Geometry: final body of the model. Coordinates: model frame, mm. A direction names the side the tool comes from. Give positions to 0.01 mm unless a question says otherwise; leave off trailing zeros. Loops run counter-clockwise (first coordinate to the right, second up) from the corner with the lowest first, then second, coordinate; pieces in that order, holes last. Notation, with made-up numbers: (3, 13.5) -> (37, 13.5) arc R26 cw to (37, 39.5) -> close; hole circle Ø8 at (25.5, -4). An arc over 180 degrees is marked (long way). One line per item, written item: value. Start each with the question number.
Autodesk Inventor part; units mm, degrees
ref_plane "YZ Plane" through (0, 0, 0) normal (1, 0, 0) x (0, 1, 0)
ref_plane "XZ Plane" through (0, 0, 0) normal (0, 1, 0) x (-1, 0, 0)
ref_plane "XY Plane" through (0, 0, 0) normal (0, 0, 1) x (1, 0, 0)
sketch "Sketch1" plane through (0, 0, 0) normal (0, 1, 0) x (-1, 0, 0)
  line L0 (0, 0) -> (80, 0)
  line L1 (80, 0) -> (80, 3.95)
  line L2 (80, 3.95) -> (67, 3.95)
  line L3 (67, 3.95) -> (67, 5)
  line L4 (67, 5) -> (62, 5)
  line L5 (62, 5) -> (62, 6)
  line L6 (62, 6) -> (18, 6)
  line L7 (18, 6) -> (18, 5)
  line L8 (18, 5) -> (13, 5)
  line L9 (13, 5) -> (13, 3.95)
  line L10 (13, 3.95) -> (0, 3.95)
  line L11 (0, 3.95) -> (0, 0)
  point P0 (40, 6)
  dimension "d0" = 80
  dimension "d1" = 3.95
  dimension "d2" = 18
  dimension "d3" = 5
  dimension "d4" = 5
  dimension "d5" = 6
  dimension "d6" = 22
  dimension "d7" = 5
revolve "Revolution1" add sketch "Sketch1" angle 360 about axis through (0, 0, 0) along (-1, 0, 0)
chamfer "Chamfer1" distance 1 angle 45 2 edges at (-80, 0, -3.95) (0, 0, -3.95)
sketch "Sketch2" plane through (0, 0, 0) normal (0, 1, 0) x (-1, 0, 0)
  circle A0 centre (77.5, 0) radius 1.2
  line L0 (80, 2.95) -> (80, -2.95)
  circle A1 centre (2.5, 0) radius 1.2
  line L1 (0, -2.95) -> (0, 2.95)
  point P0 (0, 0)
  dimension "d12" = 2.4
  dimension "d13" = 2.5
  dimension "d14" = 2.4
  dimension "d15" = 2.5
extrude "Extrusion1" cut sketch "Sketch2" along normal mid plane 10
properties part number "Axel" material "Iron, Cast"
Item 1: Section D-D, the plane x = -77.5. Output: boundary loops of the cut face in (y, z), then the cut area to 3 significant figures.
Item 2: Mould query, pull axis Z, two halves, no side actions, for faces 4 (the face through (-3.61, -0.06, 0.46)), 5 (the face through (-64.46, 4.88, -1.08)), 6 (the face through (0, 0, 0)). Classes: pulls with the +Z half, pulls with the -Z half, needs draft (parallel to the pull), parting line crosses it, or undercut.
Item 3: Pin query (flat end, axial travel): pin 1 (3 mm diameter, centred on y = 2, z = -1, fed in from +X); pin 2 (1.5 mm diameter, centred on x = -18, z = 1.5, fed in from -Y); pin 3 (4 mm diameter, centred on x = -72, z = -4.5, fed in from +Y); pin 4 (1 mm diameter, centred on x = -42, z = 1.5, fed in from +Y). Return the tip coordinate at first contact, or that it passes through.
Item 4: Access query for faces 1 (the face through (-67, 2, 4)), 2 (the face through (-13, 2, 4)), 3 (the face through (-80, 0, 0)). Directions: +Z, -Z, +X, -X, +Y, -Y. A direction counts if a zero-diameter tool reaches every point of the face in a straight line with its end or side. Return the directions, or none.
Item 5: Section C-C, the plane x = -25. Output: boundary loops of the cut face in (y, z), then the cut area to 3 significant figures.
Item 6: Section A-A, the plane z = 0. State how many separate pieces and enclosed holes the cut face has, then the cut area to 3 significant figures.
Item 7: Ray query, line 1 along X through (y, z) = (0.5, 0); line 2 along X through (y, z) = (0.5, -1); line 3 along X through (y, z) = (-4, -3.5). Return the intervals inside material, ascending. Write a range as [from, to].
Item 8: Section B-B, the plane y = 0. Output: boundary loops of the cut face in (x, z), then the cut area to 3 significant figures.
Geometry check:
1. outline: (-3.76, -1.2) arc R3.95 ccw to (3.76, -1.2) -> close; (-3.76, 1.2) -> (3.76, 1.2) arc R3.95 ccw to start
1. area: 30.4 mm2
2. face 4: undercut
2. face 5: parting line crosses it
2. face 6: needs draft
3. pin 1: stops at x = 0
3. pin 2: stops at y = -5.95
3. pin 3: stops at y = 3.06
3. pin 4: stops at y = 5.92
4. face 1: -X
4. face 2: +X
4. face 3: +Z, -Z, -X, +Y, -Y
5. outline: circle Ø12 at (0, 0)
5. area: 113 mm2
6. separate pieces: 3
6. enclosed holes: 0
6. area: 793 mm2
7. line 1: x = [-80, -78.7], [-76.3, -3.7], [-1.3, 0]
7. line 2: x = [-80, -78.16], [-76.84, -3.16], [-1.84, 0]
7. line 3: x = [-62, -18]
8. outline: (-80, -2.95) -> (-79, -3.95) -> (-67, -3.95) -> (-67, -5) -> (-62, -5) -> (-62, -6) -> (-18, -6) -> (-18, -5) -> (-13, -5) -> (-13, -3.95) -> (-1, -3.95) -> (0, -2.95) -> (0, 2.95) -> (-1, 3.95) -> (-13, 3.95) -> (-13, 5) -> (-18, 5) -> (-18, 6) -> (-62, 6) -> (-62, 5) -> (-67, 5) -> (-67, 3.95) -> (-79, 3.95) -> (-80, 2.95) -> close; hole circle Ø2.4 at (-77.5, 0); hole circle Ø2.4 at (-2.5, 0)
8. area: 822 mm2
